from build123d import *

# Parameters (mm, degrees)
SKETCH1_W           = 140
SKETCH1_H           = 150
BOSS_EXTRUDE1_DEPTH = 240
SKETCH2_R           = 65
BOSS_EXTRUDE2_DEPTH = 20
SKETCH3_R           = 75
BOSS_EXTRUDE3_DEPTH = 10
SKETCH4_R           = 40
CUT_EXTRUDE2_DEPTH  = 50
SKETCH5_R           = 50
BOSS_EXTRUDE4_DEPTH = 90
FILLET1_R           = 2
FILLET2_R           = 20
FILLET3_R           = 10
SKETCH6_R           = 65
BOSS_EXTRUDE5_DEPTH = 10
BOSS_EXTRUDE6_DEPTH = 75
CUT_EXTRUDE3_DEPTH  = 50
SKETCH9_R           = 50
BOSS_EXTRUDE7_DEPTH = 100
FILLET4_R           = 2
CUT_EXTRUDE5_DEPTH  = 2


with BuildPart() as part:
    # Sketch1 → Boss-Extrude1 (new body)
    with BuildSketch(Plane(origin=(0, 0, 0), x_dir=(1, 0, 0), z_dir=(0, 1, 0))):
        Rectangle(SKETCH1_W, SKETCH1_H)
    extrude(amount=BOSS_EXTRUDE1_DEPTH)

    # Sketch2 → Boss-Extrude2 (add)
    with BuildSketch(Plane(origin=(0, 240, 0), x_dir=(1, 0, 0), z_dir=(0, 1, 0))):
        with Locations(Location((0, 0, 0), (0, 0, 270))):
            Circle(SKETCH2_R)
    extrude(amount=BOSS_EXTRUDE2_DEPTH)

    # Sketch3 → Boss-Extrude3 (add)
    with BuildSketch(Plane(origin=(0, 260, 0), x_dir=(1, 0, 0), z_dir=(0, 1, 0))):
        with Locations(Location((0, 0, 0), (0, 0, 270))):
            Circle(SKETCH3_R)
    extrude(amount=BOSS_EXTRUDE3_DEPTH)

    # Sketch4 → Cut-Extrude2 (cut)
    with BuildSketch(Plane(origin=(0, 270, 0), x_dir=(1, 0, 0), z_dir=(0, 1, 0))):
        with Locations(Location((0, 0, 0), (0, 0, 270))):
            Circle(SKETCH4_R)
    extrude(amount=-CUT_EXTRUDE2_DEPTH, mode=Mode.SUBTRACT)

    # Sketch5 → Boss-Extrude4 (add, symmetric)
    with BuildSketch(Plane(origin=(0, 0, 0), x_dir=(0, 0, -1), z_dir=(1, 0, 0))):
        with BuildLine():
            Line((-75, 155), (-145, 155))
            ThreePointArc((-145, 155), (-214.72110169, 91.242433746), (-157.435124514, 16.113370831))
            Line((-157.435124514, 16.113370831), (-75, 0))
            Line((-75, 0), (-75, 155))
        make_face()
        with Locations(Location((-145, 85, 0), (0, 0, 180))):
            Circle(SKETCH5_R, mode=Mode.SUBTRACT)
    extrude(amount=BOSS_EXTRUDE4_DEPTH, both=True)

    # Fillet1
    fillet1_edges = [part.edges().sort_by_distance(p)[0] for p in [
        (0, 240, -65),
    ]]
    fillet(fillet1_edges, radius=FILLET1_R)

    # Fillet2
    fillet2_edges = [part.edges().sort_by_distance(p)[0] for p in [
        (-70, 77.5, 75),
        (70, 77.5, 75),
    ]]
    fillet(fillet2_edges, radius=FILLET2_R - 0.0001)  # a hair under: the kernel refuses the full size

    # Fillet3
    fillet3_edges = [part.edges().sort_by_distance(p)[0] for p in [
        (-70, 120, -75),
        (70, 120, -75),
        (70, 197.5, 75),
        (-70, 197.5, 75),
    ]]
    fillet(fillet3_edges, radius=FILLET3_R)

    # Sketch6 → Boss-Extrude5 (add)
    with BuildSketch(Plane(origin=(0, 270, 0), x_dir=(1, 0, 0), z_dir=(0, 1, 0))):
        with Locations(Location((0, 0, 0), (0, 0, 270))):
            Circle(SKETCH6_R)
    extrude(amount=BOSS_EXTRUDE5_DEPTH)

    # Sketch7 → Boss-Extrude6 (add, symmetric)
    with BuildSketch(Plane(origin=(0, 0, 0), x_dir=(0, 0, -1), z_dir=(1, 0, 0))):
        with BuildLine():
            Line((-75, 280), (75, 280))
            Line((75, 280), (75, 480))
            ThreePointArc((75, 480), (-9.573e-06, 554.999990364), (-75, 479.999980853))
            Line((-75, 479.999980853), (-75, 280))
        make_face()
    extrude(amount=BOSS_EXTRUDE6_DEPTH, both=True)

    # Sketch8 → Cut-Extrude3 (cut, symmetric)
    with BuildSketch(Plane(origin=(0, 0, 0), x_dir=(0, 0, -1), z_dir=(1, 0, 0))):
        with BuildLine():
            Line((75, 479.999980853), (75, 379.999990427))
            Line((75, 379.999990427), (-75, 379.999990427))
            Line((-75, 379.999990427), (-75, 479.999980853))
            ThreePointArc((-75, 479.999980853), (0, 554.999990364), (75, 479.999980853))
        make_face()
    extrude(amount=CUT_EXTRUDE3_DEPTH, both=True, mode=Mode.SUBTRACT)

    # Sketch9 → Boss-Extrude7 (add)
    with BuildSketch(Plane.ZY.offset(-50)):
        with Locations(Location((0, 479.999990364, 0), (0, 0, 180))):
            Circle(SKETCH9_R)
    extrude(amount=BOSS_EXTRUDE7_DEPTH)

    # Fillet4
    fillet4_edges = [part.edges().sort_by_distance(p)[0] for p in [
        (0, 280, -65),
    ]]
    fillet(fillet4_edges, radius=FILLET4_R)

    # Sketch14 → Cut-Extrude5 (cut)
    with BuildSketch(Plane(origin=(0, 0, -75), x_dir=(-1, 0, 0), z_dir=(0, 0, -1))):
        with BuildLine():
            Line((-15, 239), (-15, 189))
            ThreePointArc((-15, 189), (0, 174), (15, 189))
            Line((15, 189), (15, 239))
            Line((15, 239), (-15, 239))
        make_face()
    extrude(amount=-CUT_EXTRUDE5_DEPTH, mode=Mode.SUBTRACT)


with BuildPart() as part_1:
    # Body-Move/Copy1: moved
    add(part.part.moved(Location((0, -85, -145))))


solid = part_1.part
Could you check a few things on this model? Use its own coordinates, in mm. A direction names the side the tool comes from. Give positions to 0.01 mm unless a question says otherwise; leave off trailing zeros. Loops run counter-clockwise (first coordinate to the right, second up) from the corner with the lowest first, then second, coordinate; pieces in that order, holes last. Notation, with made-up numbers: (63.5, 32) -> (83.5, 32) arc R25 cw to (83.5, 64) -> close; hole circle Ø4 at (48.5, -28). An arc over 180 degrees is marked (long way). Return JSON: item names as keys, results as strings.
Item 1: I need wall thicknesses on L1, parallel to Z at x = -51, y = 0; L2, parallel to X at y = 174.5, z = -145; L3, parallel to X at y = 150.5, z = -145. Which ranges of each line are inside material? Lowest first, please. Write a range as from..to.
Geometry results:
{"L1": "z = -220..-50, 50..70", "L2": "x = -65..-40, 40..65", "L3": "x = -70..-40, 40..70"}
Item 2: We'd pull the mould along Z, two halves only. Please class faces 5 (the cylindrical face through (0.7, 392.8, -95.05)), 6 (the flat face through (-90, -24, -46)), 7 (the cylindrical face through (1.76, 160.35, -184.96)): +Z half, -Z half, draft (parallel to the pull), parting line (faces both ways), or undercut.
Geometry results:
{"face 5": "parting line", "face 6": "draft", "face 7": "undercut"}
Item 3: If we section it at C-C on z = -18: List the corners of the cut face in (x, y) for me, plus the area to 3 significant figures.
Geometry results:
{"outline": "(-90, -74.84) -> (90, -74.84) -> (90, -46.65) -> (-90, -46.65) -> close; (-90, 46.65) -> (90, 46.65) -> (90, 70) -> (-90, 70) -> close", "area": "9,280 mm²"}
Item 4: If we section it at B-B on x = 0: Count the separate pieces of the cut face and the enclosed holes in it, plus the area to 3 significant figures.
Geometry results:
{"separate pieces": "2", "enclosed holes": "2", "area": "70,300 mm²"}
Item 5: I'm going to push flat-ended pins straight in: pin 1 (12 mm diameter, centred on x = 50.5, z = -191, fed in from +Y); pin 2 (12 mm diameter, centred on y = 29.5, z = -88, fed in from +X); pin 3 (2 mm diameter, centred on x = -30.5, z = -9, fed in from -Y). Where does each tip first touch, or does it pass through?
Geometry results:
{"pin 1": "stops at y = 458.44", "pin 2": "stops at x = 71.67", "pin 3": "stops at y = -73.27"}
Item 6: Which directions (+Z, -Z, +X, -X, +Y, -Y) give clear straight access to the entire face, cutting with the end or side of a thin tool? Please do faces 1 (the cylindrical face through (-67.15, 113.1, -73.01)), 2 (the cylindrical face through (75.703, -6.415, -76.014)), 3 (the cylindrical face through (66.99, 113.1, -72.85)), 4 (the flat face through (1, 135, -146)).
Geometry results:
{"face 1": "+Z, -X", "face 2": "-Z, +X, -Y", "face 3": "+Z, +X", "face 4": "none"}
Item 7: If we section it at D-D on y = 389: List the corners of the cut face in (x, z) for me.
Geometry results:
{"outline": "(-75, -220) -> (-50, -220) -> (-50, -194.64) -> (50, -194.64) -> (50, -220) -> (75, -220) -> (75, -70) -> (50, -70) -> (50, -95.36) -> (-50, -95.36) -> (-50, -70) -> (-75, -70) -> close"}
